Design review of the part built by this model. Coordinates are the model's own, in mm. A direction names the side the tool comes from. Round coordinates to 2 decimals unless told otherwise and drop trailing zeros. Loops run counter-clockwise (first coordinate to the right, second up) from the corner with the lowest first, then second, coordinate; pieces in that order, holes last. Notation, with made-up numbers: (-11.5, 28) -> (34.5, 28) arc R5 ccw to (34.5, 32) -> close; hole circle Ø4 at (51.5, -17.75). An arc over 180 degrees is marked (long way). Use a Markdown table: item, result. Add a question column.
Autodesk Inventor part; units mm, degrees
ref_plane "YZ Plane" through (0, 0, 0) normal (1, 0, 0) x (0, 1, 0)
ref_plane "XZ Plane" through (0, 0, 0) normal (0, 1, 0) x (-1, 0, 0)
ref_plane "XY Plane" through (0, 0, 0) normal (0, 0, 1) x (1, 0, 0)
sketch "Sketch1" plane through (0, 0, 0) normal (0, 0, 1) x (1, 0, 0)
  line L0 (0, 0) -> (15.748, 0)
  line L1 (15.748, 0) -> (15.748, 25.4)
  line L2 (15.748, 25.4) -> (0, 25.4)
  line L3 (0, 25.4) -> (0, 0)
  line L4 (0, 0) -> (5.2493, 0)
  line L5 (5.2493, 0) -> (5.2493, -5.08)
  line L6 (5.2493, -5.08) -> (0, -5.08)
  line L7 (0, -5.08) -> (0, 0)
  line L8 (10.4987, 0) -> (15.748, 0)
  line L9 (15.748, 0) -> (15.748, -5.08)
  line L10 (15.748, -5.08) -> (10.4987, -5.08)
  line L11 (10.4987, -5.08) -> (10.4987, 0)
  dimension "d0" = 25.4
  dimension "d1" = 15.748
  dimension "d2" = 5.2493
  dimension "d3" = 5.08
  dimension "d4" = 0
  dimension "d5" = 5.2493
extrude "Extrusion1" add sketch "Sketch1" along normal blind 2.794
sketch "Sketch2" plane through (0, 0, 2.794) normal (0, 0, 1) x (1, 0, 0)
  circle A0 centre (3.048, 22.352) radius 1.651
  circle A1 centre (12.7, 3.048) radius 1.651
  line L0 (10.4987, 0) -> (10.4987, -5.08)
  line L1 (10.4987, -5.08) -> (15.748, -5.08)
  line L2 (15.748, -5.08) -> (15.748, 25.4)
  line L3 (15.748, 25.4) -> (0, 25.4)
  line L4 (0, 25.4) -> (0, -5.08)
  line L5 (0, -5.08) -> (5.2493, -5.08)
  line L6 (5.2493, -5.08) -> (5.2493, 0)
  line L7 (5.2493, 0) -> (10.4987, 0)
  line L8 (5.2493, 0) -> (10.4987, 0) construction
  line L9 (7.874, 0) -> (7.874, 25.4) construction
  line L10 (7.874, 12.7) -> (15.748, 12.7) construction
  circle A2 centre (12.7, 22.352) radius 1.651
  circle A3 centre (3.048, 3.048) radius 1.651
  point P0 (0, 0)
extrude "Extrusion2" cut sketch "Sketch2" against normal blind 25.4 contours A0 | A1 | A2 | A3
sketch "Sketch3" plane through (0, 0, 2.794) normal (0, 0, 1) x (1, 0, 0)
  circle A0 centre (12.7, 22.352) radius 1.651
  circle A1 centre (3.048, 22.352) radius 1.651
  circle A2 centre (12.7, 3.048) radius 1.651
  circle A3 centre (3.048, 3.048) radius 1.651
  line L0 (10.4987, 0) -> (10.4987, -5.08)
  line L1 (10.4987, -5.08) -> (15.748, -5.08)
  line L2 (15.748, -5.08) -> (15.748, 25.4)
  line L3 (15.748, 25.4) -> (0, 25.4)
  line L4 (0, 25.4) -> (0, -5.08)
  line L5 (0, -5.08) -> (5.2493, -5.08)
  line L6 (5.2493, -5.08) -> (5.2493, 0)
  line L7 (5.2493, 0) -> (10.4987, 0)
  line L8 (0, 0) -> (-3.81, 0)
  line L9 (-3.81, 0) -> (-3.81, 26.035)
  line L10 (-0.635, 29.21) -> (16.383, 29.21)
  line L11 (19.558, 26.035) -> (19.558, 0)
  line L12 (19.558, 0) -> (15.748, 0)
  arc A4 (-0.635, 29.21) -> (-3.81, 26.035) centre (-0.635, 26.035) ccw
  arc A5 (19.558, 26.035) -> (16.383, 29.21) centre (16.383, 26.035) ccw
  line L13 (0, 0) -> (0, 25.4)
  line L14 (15.748, 25.4) -> (0, 25.4)
  line L15 (0, 25.4) -> (15.748, 25.4)
  line L16 (15.748, 25.4) -> (15.748, 0)
  dimension "d10" = 3.81
  dimension "d11" = 3.81
  dimension "d12" = 3.81
  dimension "d13" = 3.175
extrude "Extrusion3" add sketch "Sketch3" against normal blind 2.794 contours L2 L3 L4 L8 L9 A4 L10 A5 L11 L12
equation "\"d2\" = 0.333333 * d1"
equation "\"d5\" = d2"
equation "\"d11\" = d10"
equation "\"d12\" = d11"
properties part number "LimitSwitchMount" material "Polycarbonate, Smoke"
1. Consider section A-A on x = 12.7. State the section outline as (y, z) points.
2. Insertion check: P1, Ø0.8, axis at y = -3, z = 1.5, coming from the +X side; P2, Ø0.8, axis at x = 17, z = 1, coming from the -Y side; P3, Ø1.4, axis at y = -2.5, z = 2, coming from the -X side. Each pin has a flat end and moves straight along its axis. Give the tip position at first contact, or say it passes through.
3. Consider section B-B on y = -1. State the section outline as (x, z) points, plus the area to 3 significant figures.
4. Consider section C-C on y = 21.5. State the section outline as (x, z) points.
5. For faces 1 (the face through (0, -3, 1)), 2 (the face through (18, 0, 1)), 3 (the face through (3, -5.08, 1)), 4 (the face through (8, 0, 1)), 5 (the face through (8, 12, 2.794)), list the 3-axis set-ups (+Z, -Z, +X, -X, +Y, -Y) from which the entire face can be reached by the end or side of a thin tool; tool diameter is ignored.
6. To check wall thickness, follow probe 1 along Y at (x, z) = (12.7, 0.7); probe 2 along X at (y, z) = (2.5, 2.45); probe 3 along X at (y, z) = (22, 1.6). State the ranges of each line that lie inside material, in increasing order. Write a range as from..to.
7. Consider section D-D on z = 2.2. State the section outline as (x, y) points (3 decimals).
8. Mouldability with a two-part tool opening along Y and no side actions: class faces 6 (the face through (-2, 0, 1)), 7 (the face through (10.499, -3, 1)), 8 (the face through (3.94, 23.74, 1.42)), 9 (the face through (12.342, 1.436, 1.417)) as +Y half, -Y half, draft (parallel to the pull), parting line (faces both ways), or undercut.
Verdict:
| question | item | result |
|---|---|---|
| 1 | outline | (-5.08, 0) -> (1.4, 0) -> (1.4, 2.79) -> (-5.08, 2.79) -> close; (4.7, 0) -> (20.7, 0) -> (20.7, 2.79) -> (4.7, 2.79) -> close; (24, 0) -> (29.21, 0) -> (29.21, 2.79) -> (24, 2.79) -> close |
| 2 | P1 | stops at x = 15.75 |
| 2 | P2 | stops at y = 0 |
| 2 | P3 | stops at x = 0 |
| 3 | outline | (0, 0) -> (5.25, 0) -> (5.25, 2.79) -> (0, 2.79) -> close; (10.5, 0) -> (15.75, 0) -> (15.75, 2.79) -> (10.5, 2.79) -> close |
| 3 | area | 29.3 mm² |
| 4 | outline | (-3.81, 0) -> (1.63, 0) -> (1.63, 2.79) -> (-3.81, 2.79) -> close; (4.46, 0) -> (11.29, 0) -> (11.29, 2.79) -> (4.46, 2.79) -> close; (14.11, 0) -> (19.56, 0) -> (19.56, 2.79) -> (14.11, 2.79) -> close |
| 5 | face 1 | +Z, -Z, -X, -Y |
| 5 | face 2 | +Z, -Z, +X, -Y |
| 5 | face 3 | +Z, -Z, +X, -X, -Y |
| 5 | face 4 | +Z, -Z, -Y |
| 5 | face 5 | +Z, +X, -X, +Y, -Y |
| 6 | probe 1 | y = -5.08..1.4, 4.7..20.7, 24..29.21 |
| 6 | probe 2 | x = -3.81..1.49, 4.61..11.14, 14.26..19.56 |
| 6 | probe 3 | x = -3.81..1.43, 4.66..11.09, 14.31..19.56 |
| 7 | outline | (-3.81, 0) -> (0, 0) -> (0, -5.08) -> (5.249, -5.08) -> (5.249, 0) -> (10.499, 0) -> (10.499, -5.08) -> (15.748, -5.08) -> (15.748, 0) -> (19.558, 0) -> (19.558, 26.035) arc R3.175 ccw to (16.383, 29.21) -> (-0.635, 29.21) arc R3.175 ccw to (-3.81, 26.035) -> close; hole circle Ø3.302 at (3.048, 3.048); hole circle Ø3.302 at (3.048, 22.352); hole circle Ø3.302 at (12.7, 3.048); hole circle Ø3.302 at (12.7, 22.352) |
| 8 | face 6 | -Y half |
| 8 | face 7 | draft |
| 8 | face 8 | undercut |
| 8 | face 9 | undercut |
